```python
from build123d import *

# Parameters (mm, degrees)
SKETCH_R      = 6.5
PAD_DEPTH     = 3
PAD001_DEPTH  = 25
SKETCH002_R   = 8.5
SKETCH002_R_2 = 6.5
PAD002_DEPTH  = 1
SKETCH003_R   = 7
PAD003_DEPTH  = 1
SKETCH004_R   = 3.75
PAD004_DEPTH  = 29
SKETCH005_W   = 0.25
SKETCH005_H   = 1.1
SKETCH006_R   = 1.5
POCKET_DEPTH  = 50


with BuildPart() as part:
    # Sketch → Pad (new body)
    with BuildSketch(Plane.XY):
        with BuildLine():
            ThreePointArc((-25, 30), (-55, 0), (-25, -30))
            Line((-25, -30), (25, -30))
            ThreePointArc((25, -30), (55, 0), (25, 30))
            Line((-25, 30), (25, 30))
        make_face()
        with Locations((-17.75, 0)):
            Circle(SKETCH_R, mode=Mode.SUBTRACT)
    extrude(amount=PAD_DEPTH)

    # Sketch001 (on Face7 of Pad) → Pad001 (join)
    with BuildSketch(Plane.XY.offset(3)):
        with BuildLine():
            ThreePointArc((-25, 30), (-55, 0), (-25, -30))
            Line((-25, -30), (25, -30))
            ThreePointArc((25, -30), (55, 0), (25, 30))
            Line((-25, 30), (25, 30))
        make_face()
        with BuildLine():
            ThreePointArc((-25, 25), (-50, 0), (-25, -25))
            Line((-25, -25), (25, -25))
            ThreePointArc((25, -25), (50, 0), (25, 25))
            Line((-25, 25), (25, 25))
        make_face(mode=Mode.SUBTRACT)
    extrude(amount=PAD001_DEPTH)

    # Sketch002 (on Face11 of Pad001) → Pad002 (join)
    with BuildSketch(Plane.XY.offset(3)):
        with Locations((-17.75, 0)):
            Circle(SKETCH002_R)
        with Locations((-17.75, 0)):
            Circle(SKETCH002_R_2, mode=Mode.SUBTRACT)
    extrude(amount=PAD002_DEPTH)

    # Sketch003 (on Face19 of Pad002) → Pad003 (join)
    with BuildSketch(Plane.XY.offset(3)):
        with Locations((14.25, 0)):
            Circle(SKETCH003_R)
    extrude(amount=PAD003_DEPTH)

    # Sketch004 (on Face21 of Pad003) → Pad004 (join)
    with BuildSketch(Plane.XY.offset(4)):
        with Locations((14.25, 0)):
            Circle(SKETCH004_R)
    extrude(amount=PAD004_DEPTH)

    # Sketch005 (on DatumPlane) → Groove (revolve, cut)
    with BuildSketch(Plane(origin=(14.25, 0, 18.5), x_dir=(1, 0, 0), z_dir=(0, -1, 0))):
        with Locations((3.625, 13.05)):
            Rectangle(SKETCH005_W, SKETCH005_H)
    revolve(axis=Axis((14.25, 0, 18.5), (0, 0, 1)), mode=Mode.SUBTRACT)

    # Sketch006 (on Face1 of Groove) → Pocket (cut)
    with BuildSketch(Plane(origin=(0, 0, 0), x_dir=(1, 0, 0), z_dir=(0, 0, -1))):
        with Locations((-44.445436, 19.445436)):
            Circle(SKETCH006_R)
        with Locations((44.445436, 19.445436)):
            Circle(SKETCH006_R)
        with Locations((-44.445436, -19.445436)):
            Circle(SKETCH006_R)
        with Locations((44.445436, -19.445436)):
            Circle(SKETCH006_R)
        with Locations((-25, 27.5)):
            Circle(SKETCH006_R)
        with Locations((0, 27.5)):
            Circle(SKETCH006_R)
        with Locations((25, 27.5)):
            Circle(SKETCH006_R)
        with Locations((52.5, 0)):
            Circle(SKETCH006_R)
        with Locations((25, -27.5)):
            Circle(SKETCH006_R)
        with Locations((0, -27.5)):
            Circle(SKETCH006_R)
        with Locations((-25, -27.5)):
            Circle(SKETCH006_R)
        with Locations((-52.5, 0)):
            Circle(SKETCH006_R)
    extrude(amount=-POCKET_DEPTH, mode=Mode.SUBTRACT)


solid = part.part
```
Part model, mm, in its own coordinate system. A direction names the side the tool comes from. Round coordinates to 2 decimals unless told otherwise and drop trailing zeros. Order: outer loops, then holes, each group sorted by start corner. A loop starts at its lowest first (then second) coordinate and runs counter-clockwise, first axis right, second up. Notation, with made-up numbers: M 65,88.25 L 86,88.25 A28 ccw 86,110.25 Z; hole C 12,18 d7. An arc over 180 degrees is marked long. Answer in a Markdown table with one row per item. Add a question column.
Q1. Cut at B-B on z = 11. Give the number of separate pieces and of enclosed holes in the cut face, and give its area (3 significant figures).
Q2. 3-axis set-ups, long thin cutter, end or side, ignore diameter. For faces 4 (the face through (-13.18, 7.167, 3.493)), 5 (the face through (-1, 0, 0)): which of +Z, -Z, +X, -X, +Y, -Y reach the whole face in a straight line?
Q3. Mould opens along X. For faces 1 (the face through (14, 0, 33)), 2 (the face through (-26.11, -28.51, 13.8)), 3 (the face through (49.994, -0.55, 15.325)) say: +X half, -X half, draft (parallel to the pull), parting line (faces both ways), or undercut.
Q4. Wall check: L1, parallel to Y at x = 0, z = 6; L2, parallel to Y at x = -0.5, z = 11; L3, parallel to Y at x = 13.5, z = 21.5. Give the ranges that are in metal, low to high. Write a range as from..to.
Q5. Cut at C-C on x = 14.25. Give the cut face in (y, z), and give its area (3 significant figures).
Q6. Cut at A-A on x = -17.75. Give the cut face in (y, z), and give its area (3 significant figures).
Q7. Pin check, flat tips, straight feed: pin 1 (1.8 mm diameter, centred on x = 0, y = 27.5, fed in from -Z); pin 2 (1.5 mm diameter, centred on x = -42, y = -15.5, fed in from +Z); pin 3 (5 mm diameter, centred on x = 44.45, y = 19.45, fed in from +Z); pin 4 (6 mm diameter, centred on x = -37, z = 12.5, fed in from -Y). Stop position of each tip, or through.
Q8. Cut at D-D on y = 27.5. Give the cut face in (x, z).
Established:
| question | item | result |
|---|---|---|
| 1 | separate pieces | 2 |
| 1 | enclosed holes | 13 |
| 1 | area | 1,320 mm2 |
| 2 | face 4 | +Z |
| 2 | face 5 | -Z, +X, -X, +Y, -Y |
| 3 | face 1 | draft |
| 3 | face 2 | undercut |
| 3 | face 3 | undercut |
| 4 | L1 | y = -30..-29, -26..-25, 25..26, 29..30 |
| 4 | L2 | y = -30..-28.91, -26.09..-25, 25..26.09, 28.91..30 |
| 4 | L3 | y = -30..-25, -3.67..3.67, 25..30 |
| 5 | outline | M -30,0 L 30,0 L 30,28 L 25,28 L 25,3 L 7,3 L 7,4 L 3.75,4 L 3.75,31 L 3.5,31 L 3.5,32.1 L 3.75,32.1 L 3.75,33 L -3.75,33 L -3.75,32.1 L -3.5,32.1 L -3.5,31 L -3.75,31 L -3.75,4 L -7,4 L -7,3 L -25,3 L -25,28 L -30,28 Z |
| 5 | area | 661 mm2 |
| 6 | outline | M -30,0 L -6.5,0 L -6.5,4 L -8.5,4 L -8.5,3 L -25,3 L -25,28 L -30,28 Z; M 6.5,0 L 30,0 L 30,28 L 25,28 L 25,3 L 8.5,3 L 8.5,4 L 6.5,4 Z |
| 6 | area | 395 mm2 |
| 7 | pin 1 | passes through |
| 7 | pin 2 | stops at z = 3 |
| 7 | pin 3 | stops at z = 28 |
| 7 | pin 4 | stops at y = -28.62 |
| 8 | outline | M -36.99,0 L -26.5,0 L -26.5,28 L -36.99,28 Z; M -23.5,0 L -1.5,0 L -1.5,28 L -23.5,28 Z; M 1.5,0 L 23.5,0 L 23.5,28 L 1.5,28 Z; M 26.5,0 L 36.99,0 L 36.99,28 L 26.5,28 Z |
